```python
from build123d import *

# Parameters (mm, degrees)
F1_DEPTH = 25
F3_DEPTH = 500
F4_W     = 61.7009438574
F4_H     = 57.8163862228
F4_W_2   = 65.7990336418
F4_W_3   = 62.8085494041
F4_H_2   = 69.920873642
F4_H_3   = 57.5791224837
F4_W_4   = 73.9003658295
F4_H_4   = 72.9114174843
F4_W_5   = 70.9098815918
F4_H_5   = 72.5316330791
F5_DEPTH = 450


with BuildPart() as f1:
    # F0 (on Top) → F1 (new body)
    with BuildSketch(Plane.XY):
        Polygon((1900, 0), (0, 0), (0, -600), (0, -1500), (600, -1500), (600, -600), (1900, -600), align=None)
    extrude(amount=F1_DEPTH)

    # F2 (on face) → F3 (join)
    with BuildSketch(Plane.XY.offset(25)):
        Polygon((1900, -50), (1900, 0), (0, 0), (0, -50), (0, -231.5181791782), (0, -1500), (50, -1500), (50, -50), align=None)
    extrude(amount=F3_DEPTH)

    # F4 (on face) → F5 (join)
    with BuildSketch(Plane(origin=(0, 0, 0), x_dir=(1, 0, 0), z_dir=(0, 0, -1))):
        with Locations((30.8504719287, 1471.0918068886)):
            Rectangle(F4_W, F4_H)
        with Locations((567.1004831791, 1471.0918068886)):
            Rectangle(F4_W_2, F4_H)
        with Locations((568.5957252979, 565.039563179)):
            Rectangle(F4_W_3, F4_H_2)
        with Locations((30.8504719287, 28.7895612419)):
            Rectangle(F4_W, F4_H_3)
        with Locations((1863.0498170853, 563.5442912579)):
            Rectangle(F4_W_4, F4_H_4)
        with Locations((1864.5450592041, 36.2658165395)):
            Rectangle(F4_W_5, F4_H_5)
    extrude(amount=F5_DEPTH)


solid = f1.part
```
Could you check a few things on this model? Use its own coordinates, in mm. A direction names the side the tool comes from. Give positions to 0.01 mm unless a question says otherwise; leave off trailing zeros. Loops run counter-clockwise (first coordinate to the right, second up) from the corner with the lowest first, then second, coordinate; pieces in that order, holes last. Notation, with made-up numbers: (-24.75, 81) - (-20.75, 81) arc R10 cw to (-20.75, 90) - close; hole circle Ø4 at (24, 76). An arc over 180 degrees is marked (long way). Answer in a Markdown table with one row per item. Add a question column.
Q1. Please list where these lines run through material, in increasing order: L1, parallel to Z at x = 108.5, y = -1195; L2, parallel to X at y = -1434.5, z = 127.5; L3, parallel to Y at x = 356.5, z = 64.5. Write a range as from..to.
Q2. If we section it at B-B (x = 125): List the corners of the cut face in (y, z) for me, plus the area to 3 significant figures.
Q3. For pin 1 (22 mm diameter, centred on y = -42.5, z = -334, fed in from -X); pin 2 (19.5 mm diameter, centred on x = 554, z = -218, fed in from +Y); pin 3 (3 mm diameter, centred on x = 974.5, y = -591, fed in from -Z); pin 4 (4 mm diameter, centred on x = 1177.5, y = -247.5, fed in from +Z), each with a flat end and sliding along its axis, tell me the tip position at first contact or that it passes through.
Q4. If we section it at D-D (x = 559): List the corners of the cut face in (y, z) for me.
Q5. If we section it at C-C (y = -228): List the corners of the cut face in (x, z) for me, plus the area to 3 significant figures.
Q6. We'd pull the mould along X, two halves only. Please class faces 5 (the face through (50, -785, 272)), 6 (the face through (1826.1, -563, -222)), 7 (the face through (962, -50, 272)): +X half, -X half, draft (parallel to the pull), parting line (faces both ways), or undercut.
Q7. Which directions (+Z, -Z, +X, -X, +Y, -Y) give clear straight access to the entire face, cutting with the end or side of a thin tool? Please do faces 1 (the face through (1829.09, -36, -222)), 2 (the face through (1863, -527.089, -222)), 3 (the face through (600, -1452, -143)), 4 (the face through (756, -443, 25)).
Q8. If we section it at A-A (z = -367): List the corners of the cut face in (x, y) for me, plus the area to 3 significant figures.
The answers:
| question | item | result |
|---|---|---|
| 1 | L1 | z = 0..25 |
| 1 | L2 | x = 0..50 |
| 1 | L3 | y = -50..0 |
| 2 | outline | (-1500, 0) - (0, 0) - (0, 525) - (-50, 525) - (-50, 25) - (-1500, 25) - close |
| 2 | area | 62,500 mm^2 |
| 3 | pin 1 | stops at x = 0 |
| 3 | pin 2 | stops at y = -530.08 |
| 3 | pin 3 | stops at z = 0 |
| 3 | pin 4 | stops at z = 25 |
| 4 | outline | (-1500, -450) - (-1442.18, -450) - (-1442.18, 0) - (-600, 0) - (-600, -450) - (-530.08, -450) - (-530.08, 0) - (0, 0) - (0, 525) - (-50, 525) - (-50, 25) - (-1500, 25) - close |
| 5 | outline | (0, 0) - (1900, 0) - (1900, 25) - (50, 25) - (50, 525) - (0, 525) - close |
| 5 | area | 72,500 mm^2 |
| 6 | face 5 | +X half |
| 6 | face 6 | undercut |
| 6 | face 7 | draft |
| 7 | face 1 | -Z, +Y |
| 7 | face 2 | -Z, +X, -X |
| 7 | face 3 | +Z, -Z, +X, -Y |
| 7 | face 4 | +Z, +X, -Y |
| 8 | outline | (0, -1500) - (61.7, -1500) - (61.7, -1442.18) - (0, -1442.18) - close; (0, -57.58) - (61.7, -57.58) - (61.7, 0) - (0, 0) - close; (534.2, -1500) - (600, -1500) - (600, -1442.18) - (534.2, -1442.18) - close; (537.19, -600) - (600, -600) - (600, -530.08) - (537.19, -530.08) - close; (1826.1, -600) - (1900, -600) - (1900, -527.09) - (1826.1, -527.09) - close; (1829.09, -72.53) - (1900, -72.53) - (1900, 0) - (1829.09, 0) - close |
| 8 | area | 25,800 mm^2 |
